For this review, take the finished solid that the model builds, in its own axes (mm). A direction names the side the tool comes from. Coordinates: 2 decimals unless noted, no trailing zeros. Loops run counter-clockwise (first coordinate to the right, second up) from the corner with the lowest first, then second, coordinate; pieces in that order, holes last. Notation, with made-up numbers: (0, -15.75) -> (27, -15.75) arc R28 cw to (27, 4.25) -> close; hole circle Ø7 at (40.5, 46.25). An arc over 180 degrees is marked (long way). Use a Markdown table: item, result.
from build123d import *

# Parameters (mm, degrees)
BOSS_EXTRUDE1_DEPTH = 7
BOSS_EXTRUDE2_DEPTH = 38
CUT_EXTRUDE1_DEPTH  = 48
SKETCH4_W           = 78
SKETCH4_H           = 7
BOSS_EXTRUDE3_DEPTH = 34
BOSS_EXTRUDE4_DEPTH = 7
SKETCH6_R           = 5
CUT_EXTRUDE2_DEPTH  = 21


with BuildPart() as part:
    # Sketch1 → Boss-Extrude1 (new body)
    with BuildSketch(Plane.XY):
        Polygon((39, 16.5), (-39, 52.871997336), (-39, 16.5), (-39, -16.5), (39, -16.5), align=None)
    extrude(amount=BOSS_EXTRUDE1_DEPTH)

    # Sketch2 → Boss-Extrude2 (add)
    with BuildSketch(Plane(origin=(0, 0, 0), x_dir=(-1, 0, 0), z_dir=(0, 0, -1))):
        Polygon((-29.93692213, 20.726182617), (29.93692213, 48.645814719), (32.895249962, 42.301660209), (-26.978594297, 14.382028108), align=None)
    extrude(amount=BOSS_EXTRUDE2_DEPTH)

    # Sketch3 → Cut-Extrude1 (cut)
    with BuildSketch(Plane(origin=(13.285508267, 28.490864421, 0), x_dir=(0.906307787, -0.422618262, 0), z_dir=(0.422618262, 0.906307787, 0))):
        with BuildLine():
            Line((-31.627197624, 22), (-9.689455373, 22))
            ThreePointArc((-9.689455373, 22), (7.372802376, 18), (-9.689455373, 14))
            Line((-9.689455373, 14), (-31.627197624, 14))
            ThreePointArc((-31.627197624, 14), (-35.627197624, 18), (-31.627197624, 22))
        make_face()
    extrude(amount=-CUT_EXTRUDE1_DEPTH, mode=Mode.SUBTRACT)

    # Sketch4 → Boss-Extrude3 (add)
    with BuildSketch(Plane.XY.offset(7)):
        with Locations((0, -13)):
            Rectangle(SKETCH4_W, SKETCH4_H)
    extrude(amount=BOSS_EXTRUDE3_DEPTH)

    # Sketch5 → Boss-Extrude4 (add)
    with BuildSketch(Plane.ZY.offset(39)):
        Polygon((7, -9.5), (7, 15.5), (41, -9.5), align=None)
    extrude(amount=-BOSS_EXTRUDE4_DEPTH)

    # Sketch6 → Cut-Extrude2 (cut)
    with BuildSketch(Plane(origin=(0, -9.5, 0), x_dir=(1, 0, 0), z_dir=(0, 1, 0))):
        with Locations((-19, -29)):
            Circle(SKETCH6_R)
        with Locations((19, -29)):
            Circle(SKETCH6_R)
    extrude(amount=-CUT_EXTRUDE2_DEPTH, mode=Mode.SUBTRACT)


solid = part.part
(1) Take a section at D-D on x = 16. State how many separate pieces and enclosed holes the cut face has, plus the area to 3 significant figures.
Found:
| item | result |
|---|---|
| separate pieces | 3 |
| enclosed holes | 0 |
| area | 684 mm^2 |
(2) For pin 1 Ø16 at (x, z) = (19, 29) entering from +Y; pin 2 Ø6 at (x, z) = (-19, 29) entering from +Y; pin 3 Ø3 at (y, z) = (46, -19) entering from -X; pin 4 Ø8 at (x, y) = (18.5, -2) entering from -Z, all flat-tipped, find the tip position at first contact; note any pin that passes through.
Found:
| item | result |
|---|---|
| pin 1 | stops at y = -9.5 |
| pin 2 | passes through |
| pin 3 | stops at x = -31.87 |
| pin 4 | stops at z = 0 |
(3) Mouldability with a two-part tool opening along Z and no side actions: class faces 5 (the face through (39, -11, 11)), 6 (the face through (18.503, 22.25, -18.338)), 7 (the face through (-1, 15, 7)) as pulls with the +Z half, pulls with the -Z half, needs draft (parallel to the pull), parting line crosses it, or undercut.
Found:
| item | result |
|---|---|
| face 5 | needs draft |
| face 6 | undercut |
| face 7 | pulls with the +Z half |
(4) Take a section at C-C on z = 29. Write out the cut boundary in (x, y), plus the area to 3 significant figures.
Found:
| item | result |
|---|---|
| outline | (-39, -16.5) -> (-24, -16.5) -> (-24, -9.5) -> (-32, -9.5) -> (-32, -0.68) -> (-39, -0.68) -> close; (-14, -16.5) -> (14, -16.5) -> (14, -9.5) -> (-14, -9.5) -> close; (24, -16.5) -> (39, -16.5) -> (39, -9.5) -> (24, -9.5) -> close |
| area | 468 mm^2 |
(5) Take a section at B-B on y = 9.5. Write out the cut boundary in (x, z), plus the area to 3 significant figures.
Found:
| item | result |
|---|---|
| outline | (-39, 0) -> (39, 0) -> (39, 7) -> (-32, 7) -> (-32, 15.16) -> (-39, 15.16) -> close |
| area | 603 mm^2 |
(6) For faces 1 (the face through (28.437, 17.51, -18.734)), 2 (the face through (-32, -2, 17)), 3 (the face through (-3.38, 28.54, -22.96)), 4 (the face through (-31.395, 45.518, -18.734)), list the 3-axis set-ups (+Z, -Z, +X, -X, +Y, -Y) from which the entire face can be reached by the end or side of a thin tool; tool diameter is ignored.
Found:
| item | result |
|---|---|
| face 1 | -Z, +X, -Y |
| face 2 | +Z, +X, +Y |
| face 3 | -Z, -X, -Y |
| face 4 | -Z, -X, +Y |
(7) Take a section at A-A on z = -11. Write out the cut boundary in (x, y).
Found:
| item | result |
|---|---|
| outline | (-32.9, 42.3) -> (3.73, 25.23) -> (6.68, 31.57) -> (-29.94, 48.65) -> close; (13.98, 20.44) -> (26.98, 14.38) -> (29.94, 20.73) -> (16.94, 26.79) -> close |
(8) For line 1 along X through (y, z) = (-13, 29); line 2 along Z through (x, y) = (19, -14.5); line 3 along Z through (x, y) = (-18, -3.5), list the stretches that pass through material, from the lowest coordinate up.
Found:
| item | result |
|---|---|
| line 1 | x = -39 to -24, -14 to 14, 24 to 39 |
| line 2 | z = 0 to 24, 34 to 41 |
| line 3 | z = 0 to 7 |
